```python
from build123d import *

# Parameters (mm, degrees)
CYLINDER1700_R             = 1.5
CYLINDER1700_DEPTH         = 60
CYLINDER1701_R             = 1.5
CYLINDER1701_DEPTH         = 60
CYLINDER1702_R             = 1.5
CYLINDER1702_DEPTH         = 60
CYLINDER1699_R             = 1.5
CYLINDER1699_DEPTH         = 60
CYLINDER1698_R             = 2.5
CYLINDER1698_DEPTH         = 48
BOX666_W                   = 28.8
BOX666_H                   = 34.21
BOX666_DEPTH               = 20
BOX667_W                   = 42
BOX667_H                   = 24
BOX667_DEPTH               = 24
CHAMFER038_SIZE            = 6
CHAMFER039_SIZE            = 4
CHAMFER044_SIZE            = 2
CHAMFER044_ROLL_ANGLE      = 180
CHAMFER044_PLACEMENT_ANGLE = 44.999934


with BuildPart() as obj1:
    # Cylinder1700 → Cylinder1700 (new body)
    with BuildSketch(Plane(origin=(18, 85, -57), x_dir=(1, 0, 0), z_dir=(0, 0, 1))):
        Circle(CYLINDER1700_R)
    extrude(amount=CYLINDER1700_DEPTH)


with BuildPart() as obj2:
    # Cylinder1701 → Cylinder1701 (new body)
    with BuildSketch(Plane(origin=(-18, 85, -57), x_dir=(1, 0, 0), z_dir=(0, 0, 1))):
        Circle(CYLINDER1701_R)
    extrude(amount=CYLINDER1701_DEPTH)


with BuildPart() as obj3:
    # Cylinder1702 → Cylinder1702 (new body)
    with BuildSketch(Plane(origin=(-18, 95, -57), x_dir=(1, 0, 0), z_dir=(0, 0, 1))):
        Circle(CYLINDER1702_R)
    extrude(amount=CYLINDER1702_DEPTH)


with BuildPart() as compound843:
    # Cylinder1699 → Cylinder1699 (new body)
    with BuildSketch(Plane(origin=(18, 95, -57), x_dir=(1, 0, 0), z_dir=(0, 0, 1))):
        Circle(CYLINDER1699_R)
    extrude(amount=CYLINDER1699_DEPTH)

    # Compound843: union obj1, obj2, obj3
    add(obj1.part)
    add(obj2.part)
    add(obj3.part)


with BuildPart() as compound843_1:
    # Compound843 placement: moved
    add(compound843.part.moved(Location((0, 0, -16))))


with BuildPart() as obj4:
    # Cylinder1698 → Cylinder1698 (new body)
    with BuildSketch(Plane(origin=(0, 90, -55), x_dir=(1, 0, 0), z_dir=(0, 0, 1))):
        Circle(CYLINDER1698_R)
    extrude(amount=CYLINDER1698_DEPTH)


with BuildPart() as compound805:
    # Box666 → Box666 (new body)
    with BuildSketch(Plane(origin=(-14.4, -15.34, 34), x_dir=(1, 0, 0), z_dir=(0, 0, 1))):
        with Locations((14.4, 17.105)):
            Rectangle(BOX666_W, BOX666_H)
    extrude(amount=BOX666_DEPTH)


with BuildPart() as compound805_1:
    # Compound805 placement: moved
    add(compound805.part.moved(Location((0, 90, -83))))


with BuildPart() as chamfer044:
    # Box667 → Box667 (new body)
    with BuildSketch(Plane(origin=(-21, 78, -49), x_dir=(1, 0, 0), z_dir=(0, 0, 1))):
        with Locations((21, 12)):
            Rectangle(BOX667_W, BOX667_H)
    extrude(amount=BOX667_DEPTH)

    # Cut315: cut Compound805
    add(compound805_1.part, mode=Mode.SUBTRACT)


with BuildPart() as chamfer044_1:
    # Cut315 placement: moved
    add(chamfer044.part.moved(Location((0, 0, 21))))

    # Cut316: cut obj4
    add(obj4.part, mode=Mode.SUBTRACT)

    # Chamfer038
    chamfer038_edges = [chamfer044_1.edges().sort_by_distance(p)[0] for p in [
        (-14.4, 78, -18),
        (14.4, 78, -18),
    ]]
    chamfer(chamfer038_edges, length=CHAMFER038_SIZE)

    # Cut325: cut Compound843
    add(compound843_1.part, mode=Mode.SUBTRACT)

    # Chamfer039
    chamfer039_edges = [chamfer044_1.edges().sort_by_distance(p)[0] for p in [
        (-21, 90, -4),
        (21, 90, -4),
    ]]
    chamfer(chamfer039_edges, length=CHAMFER039_SIZE)

    # Chamfer044
    chamfer044_edges = [chamfer044_1.edges().sort_by_distance(p)[0] for p in [
        (-21, 102, -18),
        (21, 102, -18),
    ]]
    chamfer(chamfer044_edges, length=CHAMFER044_SIZE)


with BuildPart() as chamfer044_2:
    # Chamfer044 roll: moved
    add(chamfer044_1.part.rotate(Axis((0, 0, 0), (1, 0, 0)), CHAMFER044_ROLL_ANGLE))


with BuildPart() as chamfer044_3:
    # Chamfer044 placement: moved
    add(chamfer044_2.part.moved(Location((0, 0, 31))).rotate(Axis((0, 0, 31), (0, 0, 1)), CHAMFER044_PLACEMENT_ANGLE))


solid = chamfer044_3.part
```
Geometry check sheet. Reference: the model listing, model coordinates, mm. A direction names the side the tool comes from. Give positions to 0.01 mm unless a question says otherwise; leave off trailing zeros. Write each loop counter-clockwise with the first axis right and the second up, starting at its lowest first coordinate (ties: lowest second). Pieces come first, ordered by that corner, then holes.
1) Gauge pin test, flat ends, axial feed: pin 1 (2.5 mm diameter, centred on x = 45, z = 48.5, fed in from +Y); pin 2 (5 mm diameter, centred on y = -76.5, z = 46.5, fed in from +X); pin 3 (4 mm diameter, centred on x = 63.64, y = -63.64, fed in from +Z). Record the tip position at first contact, or that the pin passes through.
2) Section check B-B, the plane z = 46.5. Record the boundary of the cut face in (x, y) (3 decimals).
3) Section check D-D, the plane x = 76. Record the boundary of the cut face in (y, z).
4) Section check A-A, the plane z = 42.5. Record the boundary of the cut face in (x, y) (3 decimals).
5) Release check for a two-part mould opening along X. For faces 5 (the flat face through (80, -54, 44)), 6 (the flat face through (51, -76, 59)), 7 (the flat face through (77.7, -48, 49.1)) record: pulls with the +X half, pulls with the -X half, needs draft (parallel to the pull), parting line crosses it, or undercut.
6) Material ranges on L1, parallel to Y at x = 74, z = 56.75; L2, parallel to Z at x = 69, y = -57.5; L3, parallel to Y at x = 79, z = 52.5, recorded low to high.
7) Access from +Z, -Z, +X, -X, +Y, -Y to the whole of each face (thin tool, end or side, straight path). Record for faces 1 (the cylindrical face through (55.021, -78.517, 51.605)), 2 (the flat face through (55.085, -55.224, 37.278)), 3 (the flat face through (55.489, -75.854, 49.14)), 4 (the flat face through (75.854, -55.49, 49.14)).
8) Section check C-C, the plane y = -44.5. Record the boundary of the cut face in (x, z), and give its area (3 significant figures).
Computed:
1. pin 1: stops at y = -69.58
1. pin 2: stops at x = 58.64
1. pin 3: stops at z = 38
2. outline: (40.305, -70.004) - (55.861, -85.56) - (58.69, -85.56) - (61.942, -82.307) - (49.215, -69.579) - (40.729, -69.579) - close; (69.579, -49.215) - (82.307, -61.943) - (85.56, -58.69) - (85.56, -55.862) - (70.004, -40.305) - (69.579, -40.729) - close; hole circle Ø3 at (47.376, -72.832); hole circle Ø3 at (54.447, -79.903); hole circle Ø3 at (72.832, -47.376); hole circle Ø3 at (79.903, -54.447)
3. outline: (-68.25, 35) - (-51.96, 35) - (-46.3, 39) - (-46.3, 59) - (-55.64, 59) - (-55.64, 39) - (-68.25, 39) - close
4. outline: (40.305, -70.004) - (55.861, -85.56) - (58.69, -85.56) - (61.942, -82.307) - (49.215, -69.579) - (40.729, -69.579) - close; (69.579, -49.215) - (82.307, -61.943) - (85.56, -58.69) - (85.56, -55.862) - (70.004, -40.305) - (69.579, -40.729) - close
5. face 5: undercut
5. face 6: needs draft
5. face 7: pulls with the +X half
6. L1: y = -53.64 to -48.32, -46.44 to -44.3
6. L2: z = 35 to 39
6. L3: y = -58.64 to -55.65, -53.25 to -49.3
7. face 1: +Z
7. face 2: +Z, -Z, -X, +Y
7. face 3: +Z, +X, +Y
7. face 4: +Z, -X, -Y
8. outline: (65.81, 35) - (68.54, 35) - (74.2, 39) - (74.2, 59) - (69.58, 59) - (69.58, 39) - (65.81, 39) - close
8. area: 115 mm2
